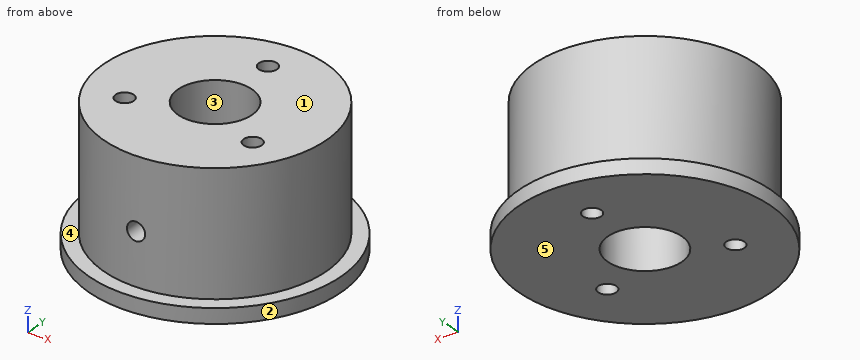
Autodesk Inventor part; units mm, degrees
ref_plane "YZ Plane" through (0, 0, 0) normal (1, 0, 0) x (0, 1, 0)
ref_plane "XY Plane" through (0, 0, 0) normal (0, 0, 1) x (1, 0, 0)
sketch "Sketch1" plane through (0, 0, 0) normal (0, 1, 0) x (-1, 0, 0)
  line L0 (0, 0) -> (0, 34.0434)
  line L1 (5, 0) -> (5, 18.5)
  line L2 (5, 18.5) -> (15, 18.5)
  line L3 (15, 18.5) -> (15, 2)
  line L4 (15, 2) -> (17, 2)
  line L5 (17, 2) -> (17, 0)
  line L6 (17, 0) -> (5, 0)
  dimension "d0" = 10
  dimension "d1" = 2
  dimension "d2" = 2
  dimension "d3" = 30
  dimension "d4" = 16.5
revolve "Revolution1" add sketch "Sketch1" angle 360 about axis through (0, 0, 0) along (0, 0, 1)
sketch "Sketch2" plane through (0, 0, 18.5) normal (0, 0, 1) x (1, 0, 0)
  circle A0 centre (0, 0) radius 5
  circle A1 centre (0, 0) radius 15
  circle A2 centre (0, 0) radius 5
  line L0 (0, 5) -> (0, 15)
  point P0 (0, 10)
  point P1 (0, 10)
  point P2 (-8.6603, -5)
  point P3 (8.6603, -5)
  dimension "d8" = 360
hole "Hole1" at (0, 10, 18.5) at (-8.6603, -5, 18.5) at (8.6603, -5, 18.5) direction (0, 0, -1) diameter 2.459 end through all
ref_plane "Work Plane2" through (0, -15, 10.25) normal (0, 1, 0) x (-1, 0, 0)
sketch "Sketch3" plane through (0, -15, 10.25) normal (0, 1, 0) x (-1, 0, 0)
  line L0 (17, -10.25) -> (-17, -10.25)
  point P0 (0, -10.25)
  point P1 (0, -1.25)
  point P2 (0, -10.25)
  dimension "d17" = 9
hole "Hole2" at (0, -15, 9) direction (0, 1, 0) diameter 2.459 depth 12 tip angle 118
properties part number "ReelMotorBearingShaft" material "Aluminum 6061"
Here's how the part is built. I have some questions about the finished solid (model axes, mm). Face numbers are marked on the shaded views. A direction names the side the tool comes from. Give positions to 0.01 mm unless a question says otherwise; leave off trailing zeros. Write each loop counter-clockwise with the first axis right and the second up, starting at its lowest first coordinate (ties: lowest second). Pieces come first, ordered by that corner, then holes. Notation, with made-up numbers: M 31.25,-3.75 L 57.25,-3.75 A16 ccw 57.25,5.25 Z; hole C 42.5,-1 d4. An arc over 180 degrees is marked long. Put each result on its own line as item: value. Start each with the question number.
Item 1: Will these pins go through, and if not, where does the flat tip stop? pin 1 (2 mm diameter, centred on x = 7, z = 10.5, fed in from +Y); pin 2 (4 mm diameter, centred on x = 4.5, z = 6, fed in from -Y); pin 3 (1.5 mm diameter, centred on x = 0, z = 9, fed in from +Y); pin 4 (1 mm diameter, centred on x = -10.5, y = 8.5, fed in from -Z).
Item 2: On a 3-axis mill with a long thin cutter (end or side, diameter ignored), from which of +Z, -Z, +X, -X, +Y, -Y can I reach the whole of each face in a straight line? I mean the marked faces 4 and 5. Say none if no direction works.
Item 3: Thinking about a two-plate mould opening in X: for the marked faces 1, 2 and 3, which applies, +X half, -X half, draft (parallel to the pull), parting line (faces both ways), or undercut?
Item 4: If we section it at C-C, the plane z = 11.5: Write out the boundary of the cut face in (x, y).
Item 5: If we section it at D-D, the plane x = 3.5: Write out the boundary of the cut face in (y, z), then the cut area to 3 significant figures.
Item 6: If we section it at A-A, the plane y = 0: Write out the boundary of the cut face in (x, z), then the cut area to 3 significant figures.
Item 7: I need wall thicknesses on L1, parallel to X at y = -5, z = 10; L2, parallel to Y at x = 0, z = 13.75; L3, parallel to Z at x = 2.5, y = 15. Which ranges of each line are inside material? Lowest first, please. Write a range as from..to.
Item 8: If we section it at B-B, the plane x = 0: Write out the boundary of the cut face in (y, z).
Values:
1. pin 1: y = 13.75
1. pin 2: y = -14.79
1. pin 3: y = 15
1. pin 4: z = 0
2. face 4: +Z
2. face 5: -Z, +X, -X, +Y, -Y
3. face 1: draft
3. face 2: parting line
3. face 3: undercut
4. outline: C 0,0 d30; hole C -8.66,-5 d2.46; hole C 0,0 d10; hole C 0,10 d2.46; hole C 8.66,-5 d2.46
5. outline: M -16.64,0 L -3.57,0 L -3.57,18.5 L -14.59,18.5 L -14.59,2 L -16.64,2 Z; M 3.57,0 L 16.64,0 L 16.64,2 L 14.59,2 L 14.59,18.5 L 3.57,18.5 Z
5. area: 416 mm²
6. outline: M -17,0 L -5,0 L -5,18.5 L -15,18.5 L -15,2 L -17,2 Z; M 5,0 L 17,0 L 17,2 L 15,2 L 15,18.5 L 5,18.5 Z
6. area: 378 mm²
7. L1: -14.14..-9.89, -7.43..-0.72, 0.72..7.43, 9.89..14.14
7. L2: -15..-5, 5..8.77, 11.23..15
7. L3: 0..2
8. outline: M -17,0 L -5,0 L -5,7.77 L -15,7.77 L -15,2 L -17,2 Z; M -15,10.23 L -5,10.23 L -5,18.5 L -15,18.5 Z; M 5,0 L 8.77,0 L 8.77,18.5 L 5,18.5 Z; M 11.23,0 L 17,0 L 17,2 L 15,2 L 15,18.5 L 11.23,18.5 Z
